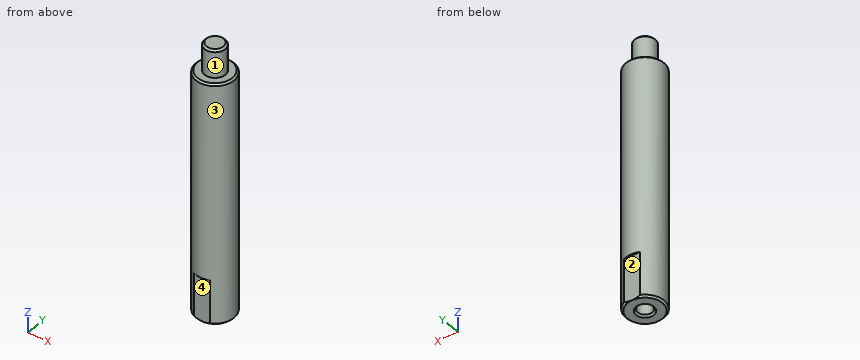
```python
from build123d import *

# Parameters (mm, degrees)
SKETCH_1_R             = 5.5
EXTRUDE_1_DEPTH        = 70
CHAMFER_1_SIZE         = 0.5
SKETCH_2_R             = 3.3
EXTRUDE_2_DEPTH        = 8
HOLE_WIZARD_M5_1_D     = 4.2
HOLE_WIZARD_M5_1_DEPTH = 12.4
HOLE_WIZARD_M5_1_TIP   = 1.2618073
CHAMFER_3_SIZE         = 0.5
SKETCH_6_W             = 10
SKETCH_6_H             = 3
CUT_EXTRUDE_1_DEPTH    = 13


# Read off the part's stored shape, not the designer's step: M6 机械螺纹 螺柱1
with BuildPart() as part:
    # 草图1 → 拉伸1 (new body)
    with BuildSketch(Plane.XY):
        Circle(SKETCH_1_R)
    extrude(amount=EXTRUDE_1_DEPTH)

    # 倒角1
    chamfer_1_edges = [part.edges().sort_by_distance(p)[0] for p in [
        (-5.5, 0, 0),
        (-5.5, 0, 70),
    ]]
    chamfer(chamfer_1_edges, length=CHAMFER_1_SIZE)

    # 草图2 → 拉伸2 (add)
    with BuildSketch(Plane.XY.offset(70)):
        Circle(SKETCH_2_R)
    extrude(amount=EXTRUDE_2_DEPTH)

    # M5 螺纹孔1
    with Locations(Plane(origin=(0, 0, 0), x_dir=(-1, 0, 0), z_dir=(0, 0, -1))):
        with Locations((0, 0)):
            Hole(HOLE_WIZARD_M5_1_D / 2, depth=HOLE_WIZARD_M5_1_DEPTH)
            with Locations((0, 0, -(HOLE_WIZARD_M5_1_DEPTH + HOLE_WIZARD_M5_1_TIP / 2))):  # 118° drill point
                Cone(0, HOLE_WIZARD_M5_1_D / 2, HOLE_WIZARD_M5_1_TIP, mode=Mode.SUBTRACT)

    # 倒角3
    chamfer_3_edges = [part.edges().sort_by_distance(p)[0] for p in [
        (-2.1, 0, 0),
    ]]
    chamfer(chamfer_3_edges, length=CHAMFER_3_SIZE)

    # 草图6 → 切除-拉伸1 (cut)
    with BuildSketch(Plane(origin=(0, 0, 0), x_dir=(-1, 0, 0), z_dir=(0, 0, -1))):
        with Locations((0, 6.5)):
            Rectangle(SKETCH_6_W, SKETCH_6_H)
        with Locations((0, -6.5)):
            Rectangle(SKETCH_6_W, SKETCH_6_H)
    extrude(amount=-CUT_EXTRUDE_1_DEPTH, mode=Mode.SUBTRACT)

    # M6 机械螺纹 螺柱1 outline → M6 机械螺纹 螺柱1 (revolve, cut)
    with BuildSketch(Plane.XZ):
        Polygon((3.3, 78), (2.4585, 78), (3, 77.4585), (3, 70), (3.3, 70), align=None)
    revolve(axis=Axis((0, 0, 0), (0, 0, 1)), mode=Mode.SUBTRACT)


solid = part.part
```
Read the model definition and answer for the solid it produces. Units are mm, in the model's axes. Face numbers are marked on the shaded views. A direction names the side the tool comes from. Coordinates: 2 decimals unless noted, no trailing zeros. Loops run counter-clockwise (first coordinate to the right, second up) from the corner with the lowest first, then second, coordinate; pieces in that order, holes last. Notation, with made-up numbers: (-8, 84) - (5, 84) arc R34 cw to (5, 120) - close; hole circle Ø3 at (37.5, 10). An arc over 180 degrees is marked (long way). Answer in a Markdown table with one row per item.
1. Given pin 1 (2.5 mm diameter, centred on x = -1, z = 6.5, fed in from -Y); pin 2 (5 mm diameter, centred on x = 1, z = 5.5, fed in from +Y); pin 3 (4 mm diameter, centred on x = 0, y = -4.5, fed in from +Z), each flat-ended and moving along its own axis, determine where each tip first touches the part or whether it passes through.
Conclusion:
| item | result |
|---|---|
| pin 1 | stops at y = -5 |
| pin 2 | stops at y = 5 |
| pin 3 | stops at z = 77.96 |
2. Straight lines are drawn through the part: line 1 (X direction, y = 0, z = 4.25); line 2 (Y direction, x = 0, z = 10); line 3 (Z direction, x = 0, y = -4.5). For each, find the intervals that lie inside material, in ascending order.
Conclusion:
| item | result |
|---|---|
| line 1 | x = -5.5 to -2.1, 2.1 to 5.5 |
| line 2 | y = -5 to -2.1, 2.1 to 5 |
| line 3 | z = 0 to 70 |
3. Find section A-A, the plane z = 26. Write down the section's boundary in (x, y), then the cut area to 3 significant figures.
Conclusion:
| item | result |
|---|---|
| outline | circle Ø11 at (0, 0) |
| area | 95.0 mm² |
4. Which of the six approach directions +Z, -Z, +X, -X, +Y, -Y give full straight-line access (tool end or side, diameter ignored) to the marked faces 1, 2, 3 and 4?
Conclusion:
| item | result |
|---|---|
| face 1 | +Z |
| face 2 | -Z, +X, -X, +Y |
| face 3 | +Z, -Z |
| face 4 | -Z, +X, -X, -Y |
